Build history of the part. All positions in model axes, mm. Face numbers are marked on the shaded views. A direction names the side the tool comes from. Round coordinates to 2 decimals unless told otherwise and drop trailing zeros. Loops run counter-clockwise (first coordinate to the right, second up) from the corner with the lowest first, then second, coordinate; pieces in that order, holes last. Notation, with made-up numbers: (0.25, 53.5) - (44.25, 53.5) arc R14 ccw to (44.25, 60.5) - close; hole circle Ø8 at (-34.75, 77.5). An arc over 180 degrees is marked (long way). Use a Markdown table: item, result.
from build123d import *

# Parameters (mm, degrees)
F0_W     = 97.8
F0_H     = 115.8
F1_DEPTH = 24.8
F2_W     = 47.4
F2_H     = 27.7
F2_H_2   = 56.4
F2_H_3   = 18.133334
F2_H_4   = 18.133333
F3_DEPTH = 23.8


with BuildPart() as f1:
    # F0 (on Top) → F1 (new body)
    with BuildSketch(Plane.XY):
        with Locations((-2.762959, -1.491597)):
            Rectangle(F0_W, F0_H)
    extrude(amount=F1_DEPTH)

    # F2 (on face) → F3 (cut)
    with BuildSketch(Plane.XY.offset(24.8)):
        with Locations((-26.962959, -44.541597)):
            Rectangle(F2_W, F2_H)
        with Locations((-26.962959, -15.841597)):
            Rectangle(F2_W, F2_H)
        with Locations((21.437041, -30.191597)):
            Rectangle(F2_W, F2_H_2)
        with Locations((21.437041, 8.07507)):
            Rectangle(F2_W, F2_H_3)
        with Locations((-26.962959, 8.07507)):
            Rectangle(F2_W, F2_H_3)
        with Locations((-26.962959, 27.208403)):
            Rectangle(F2_W, F2_H_4)
        with Locations((21.437041, 27.208403)):
            Rectangle(F2_W, F2_H_4)
        with Locations((21.437041, 46.341736)):
            Rectangle(F2_W, F2_H_4)
        with Locations((-26.962959, 46.341736)):
            Rectangle(F2_W, F2_H_4)
    extrude(amount=-F3_DEPTH, mode=Mode.SUBTRACT)


solid = f1.part
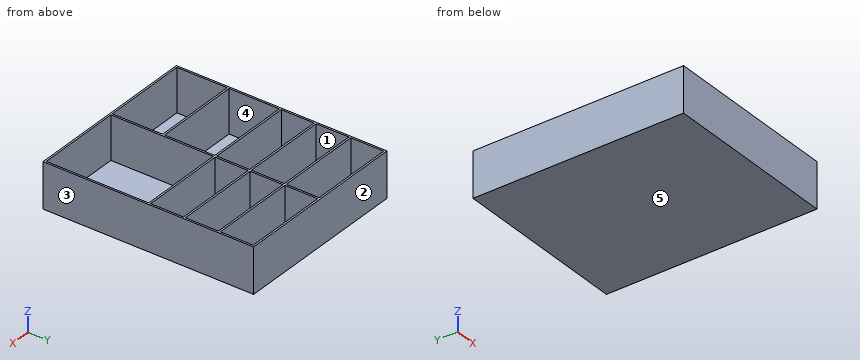
Q1. Cut at D-D, the plane x = -25. List the corners of the cut face in (y, z).
Results found:
| item | result |
|---|---|
| outline | (-59.39, 0) - (56.41, 0) - (56.41, 24.8) - (55.41, 24.8) - (55.41, 1) - (37.28, 1) - (37.28, 24.8) - (36.28, 24.8) - (36.28, 1) - (18.14, 1) - (18.14, 24.8) - (17.14, 24.8) - (17.14, 1) - (-0.99, 1) - (-0.99, 24.8) - (-1.99, 24.8) - (-1.99, 1) - (-29.69, 1) - (-29.69, 24.8) - (-30.69, 24.8) - (-30.69, 1) - (-58.39, 1) - (-58.39, 24.8) - (-59.39, 24.8) - close |
Q2. Cut at C-C, the plane z = 10.75. Count the separate pieces of the cut face and the enclosed holes in it, plus the area to 3 significant figures.
Results found:
| item | result |
|---|---|
| separate pieces | 1 |
| enclosed holes | 9 |
| area | 869 mm2 |
Q3. Drop a flat-ended pin along its axis: pin 1 (8.5 mm diameter, centred on x = -27, y = -43.5, fed in from +Z). Give the stop position or say it passes through.
Results found:
| item | result |
|---|---|
| pin 1 | stops at z = 1 |
Q4. Pull direction X, two halves, no side cores. Call the marked faces 1, 2 and 3: pulls with the +X half, pulls with the -X half, needs draft (parallel to the pull), parting line crosses it, or undercut.
Results found:
| item | result |
|---|---|
| face 1 | undercut |
| face 2 | needs draft |
| face 3 | pulls with the +X half |
Q5. Probe line 1 (X direction, y = 38.5, z = 17.5); line 2 (Y direction, x = -37.5, z = 23); line 3 (Y direction, x = 34, z = 7.5). List the from-to ranges inside material, lowest first.
Results found:
| item | result |
|---|---|
| line 1 | x = -51.66 to -50.66, -3.26 to -2.26, 45.14 to 46.14 |
| line 2 | y = -59.39 to -58.39, -30.69 to -29.69, -1.99 to -0.99, 17.14 to 18.14, 36.28 to 37.28, 55.41 to 56.41 |
| line 3 | y = -59.39 to -58.39, -1.99 to -0.99, 17.14 to 18.14, 36.28 to 37.28, 55.41 to 56.41 |
Q6. Cut at A-A, the plane x = 17.5. List the corners of the cut face in (y, z), plus the area to 3 significant figures.
Results found:
| item | result |
|---|---|
| outline | (-59.39, 0) - (56.41, 0) - (56.41, 24.8) - (55.41, 24.8) - (55.41, 1) - (37.28, 1) - (37.28, 24.8) - (36.28, 24.8) - (36.28, 1) - (18.14, 1) - (18.14, 24.8) - (17.14, 24.8) - (17.14, 1) - (-0.99, 1) - (-0.99, 24.8) - (-1.99, 24.8) - (-1.99, 1) - (-58.39, 1) - (-58.39, 24.8) - (-59.39, 24.8) - close |
| area | 235 mm2 |
Q7. Cut at B-B, the plane y = 39.5. List the corners of the cut face in (x, z).
Results found:
| item | result |
|---|---|
| outline | (-51.66, 0) - (46.14, 0) - (46.14, 24.8) - (45.14, 24.8) - (45.14, 1) - (-2.26, 1) - (-2.26, 24.8) - (-3.26, 24.8) - (-3.26, 1) - (-50.66, 1) - (-50.66, 24.8) - (-51.66, 24.8) - close |
Q8. Which spindle directions (+Z, -Z, +X, -X, +Y, -Y) get a long thin tool onto all of the face, cutting with end or side? Do the marked faces 4 and 5. Say none if no direction does.
Results found:
| item | result |
|---|---|
| face 4 | +Z |
| face 5 | -Z, +X, -X, +Y, -Y |
